Build history of the part. All positions in model axes, mm. Round coordinates to 2 decimals unless told otherwise and drop trailing zeros. Write each loop counter-clockwise with the first axis right and the second up, starting at its lowest first coordinate (ties: lowest second). Pieces come first, ordered by that corner, then holes.
1) Wall check: probe 1 along X at (y, z) = (-19, 20.5); probe 2 along X at (y, z) = (23, -165); probe 3 along Y at (x, z) = (9.25, 75). Give the ranges that are in metal, low to high.
2) Saw through at A-A (y = 7). Write the cut outline in (x, z), plus the area to 3 significant figures.
3) Saw through at B-B (z = -178). Write the cut outline in (x, y), plus the area to 3 significant figures.
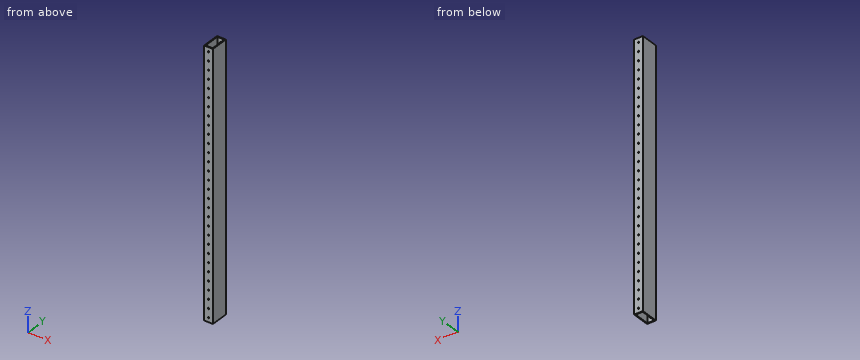
from build123d import *

# Parameters (mm, degrees)
SKETCH1_W           = 25.4
SKETCH1_H           = 50.8
SKETCH1_W_2         = 20.32
SKETCH1_H_2         = 45.72
EXTRUDE_THIN1_DEPTH = 381
SKETCH2_R           = 2.0701
CUT_EXTRUDE1_DEPTH  = 51.8
LPATTERN1_COUNT     = 31
LPATTERN1_PITCH     = 25.4


with BuildPart() as part:
    # Sketch1 → Extrude-Thin1 (new body, symmetric)
    with BuildSketch(Plane.XY):
        Rectangle(SKETCH1_W, SKETCH1_H)
        Rectangle(SKETCH1_W_2, SKETCH1_H_2, mode=Mode.SUBTRACT)
    extrude(amount=EXTRUDE_THIN1_DEPTH, both=True)

    # Sketch2 → Cut-Extrude1 (cut, through all)
    with BuildSketch(Plane(origin=(0, 25.4, 0), x_dir=(1, 0, 0), z_dir=(0, 1, 0))):
        with Locations((0, -368.3)):
            Circle(SKETCH2_R)
    cut_extrude1 = extrude(amount=-CUT_EXTRUDE1_DEPTH, mode=Mode.SUBTRACT)

    # LPattern1: Cut-Extrude1 ×31
    with Locations(*[(0, 0, -i * LPATTERN1_PITCH) for i in range(1, LPATTERN1_COUNT)]):
        add(cut_extrude1, mode=Mode.SUBTRACT)


solid = part.part
Evaluation:
1. probe 1: x = -12.7 to -10.16, 10.16 to 12.7
1. probe 2: x = -12.7 to -2.07, 2.07 to 12.7
1. probe 3: y = -25.4 to -22.86, 22.86 to 25.4
2. outline: (-12.7, -381) - (-10.16, -381) - (-10.16, 381) - (-12.7, 381) - close; (10.16, -381) - (12.7, -381) - (12.7, 381) - (10.16, 381) - close
2. area: 3,870 mm2
3. outline: (-12.7, -25.4) - (12.7, -25.4) - (12.7, 25.4) - (-12.7, 25.4) - close; hole (-10.16, -22.86) - (10.16, -22.86) - (10.16, 22.86) - (-10.16, 22.86) - close
3. area: 361 mm2
